The listing builds one solid part. Answer for the finished solid, in the listing's coordinates (mm). A direction names the side the tool comes from. Round coordinates to 2 decimals unless told otherwise and drop trailing zeros. Loops run counter-clockwise (first coordinate to the right, second up) from the corner with the lowest first, then second, coordinate; pieces in that order, holes last. Notation, with made-up numbers: (64, 51.5) - (115, 51.5) arc R16 ccw to (115, 61.5) - close; hole circle Ø7 at (41, -20.75). An arc over 180 degrees is marked (long way). One line per item, written item: value.
```python
from build123d import *

# Parameters (mm, degrees)
PAD_DEPTH            = 82.5
SKETCH001_W          = 25
SKETCH001_H          = 20
POCKET_DEPTH         = 100.001
POCKET_DEPTH_BACK    = -5.001
SKETCH002_R          = 15
POCKET001_DEPTH      = 82.501
POCKET001_DEPTH_BACK = -5.001


with BuildPart() as part:
    # Sketch → Pad (new body, symmetric)
    with BuildSketch(Plane.XZ):
        with BuildLine():
            Line((-82.5, 0), (-5, 0))
            ThreePointArc((0, -5), (-1.464466, -1.464466), (-5, 0))
            Line((0, -5), (0, -100))
            Line((5, -100), (0, -100))
            Line((5, 0), (5, -100))
            ThreePointArc((5, 0), (3.535534, 3.535534), (0, 5))
            Line((-82.5, 5), (0, 5))
            Line((-82.5, 0), (-82.5, 5))
        make_face()
    extrude(amount=PAD_DEPTH, both=True)

    # Sketch001 → Pocket (cut, two sides)
    with BuildSketch(Plane.XY) as pocket_sk:
        with Locations((-80, 28.5)):
            Rectangle(SKETCH001_W, SKETCH001_H)
    extrude(amount=-POCKET_DEPTH, mode=Mode.SUBTRACT)
    extrude(pocket_sk.sketch, amount=-POCKET_DEPTH_BACK, mode=Mode.SUBTRACT)

    # Sketch002 → Pocket001 (cut, two sides)
    with BuildSketch(Plane.YZ) as pocket001_sk:
        with Locations((-48.65, -80)):
            Circle(SKETCH002_R)
        with Locations((48.65, -80)):
            Circle(SKETCH002_R)
    extrude(amount=-POCKET001_DEPTH, mode=Mode.SUBTRACT)
    extrude(pocket001_sk.sketch, amount=-POCKET001_DEPTH_BACK, mode=Mode.SUBTRACT)


solid = part.part
```
1) For faces 1 (the flat face through (0, -1, -52)), 2 (the flat face through (-75, 18.5, 2)), 3 (the flat face through (-82.5, 60, 2)), determine the directions among +Z, -Z, +X, -X, +Y, -Y from which every point of the face is accessible in a straight line to the end or side of a thin tool.
Final values:
face 1: -Z, -X, +Y, -Y
face 2: +Z, -Z, -X
face 3: +Z, -Z, -X, +Y, -Y
2) A cutting plane is placed at B-B on z = -80. Give the vertices of the cut face in (x, y).
Final values:
outline: (0, -82.5) - (5, -82.5) - (5, -63.65) - (0, -63.65) - close; (0, -33.65) - (5, -33.65) - (5, 33.65) - (0, 33.65) - close; (0, 63.65) - (5, 63.65) - (5, 82.5) - (0, 82.5) - close
3) A cutting plane is placed at C-C on y = -14.5. Give the vertices of the cut face in (x, z).
Final values:
outline: (-82.5, 0) - (-5, 0) arc R5 cw to (0, -5) - (0, -100) - (5, -100) - (5, 0) arc R5 ccw to (0, 5) - (-82.5, 5) - close
4) A cutting plane is placed at A-A on y = -48.65. Give the vertices of the cut face in (x, z).
Final values:
outline: (-82.5, 0) - (-5, 0) arc R5 cw to (0, -5) - (0, -65) - (5, -65) - (5, 0) arc R5 ccw to (0, 5) - (-82.5, 5) - close; (0, -100) - (5, -100) - (5, -95) - (0, -95) - close
5) For a pull along Z with two mould halves and no side action, classify faces 4 (the cylindrical face through (4, -1, 3)), 5 (the cylindrical face through (2.46, -41.73, -93.31)), 6 (the flat face through (3, -1, -100)) as released by +Z, released by -Z, zero draft, split by the parting line, or undercut.
Final values:
face 4: released by +Z
face 5: undercut
face 6: released by -Z
6) A cutting plane is placed at D-D on x = -48.5. Give the vertices of the cut face in (y, z).
Final values:
outline: (-82.5, 0) - (82.5, 0) - (82.5, 5) - (-82.5, 5) - close
7) Consider L1, parallel to Y at x = 2.85, z = -80; L2, parallel to X at y = 0, z = -7. Determine where each line is inside the solid, lowest interval first.
Final values:
L1: -82.5 to -63.65, -33.65 to 33.65, 63.65 to 82.5
L2: 0 to 5
8) Each of these flat-tipped pins is pushed along its axis until it touches: pin 1 Ø1 at (y, z) = (39.5, -32) entering from -X; pin 2 Ø8 at (x, y) = (-27, 63) entering from -Z; pin 3 Ø1.5 at (y, z) = (28.5, 2) entering from -X. Where does it stop, or does it pass through?
Final values:
pin 1: x = 0
pin 2: z = 0
pin 3: x = -67.5
